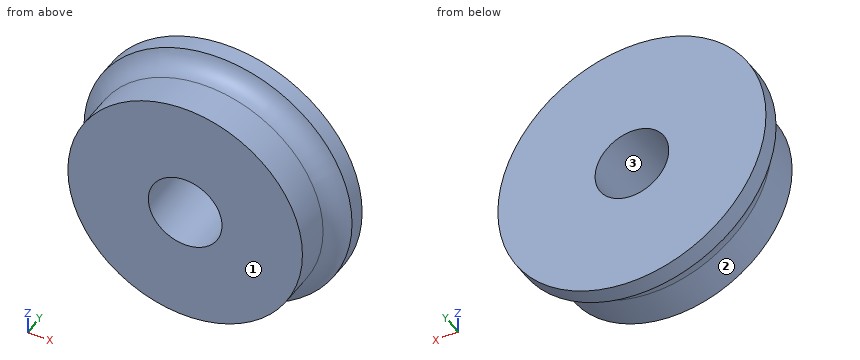
Autodesk Inventor part; units mm, degrees
ref_plane "YZ Plane" through (0, 0, 0) normal (1, 0, 0) x (0, 1, 0)
ref_plane "XZ Plane" through (0, 0, 0) normal (0, 1, 0) x (-1, 0, 0)
ref_plane "XY Plane" through (0, 0, 0) normal (0, 0, 1) x (1, 0, 0)
sketch "Boceto1" plane through (0, 0, 0) normal (0, 1, 0) x (-1, 0, 0)
  circle A0 centre (0, 0) radius 5.25
  dimension "d0" = 10.5
extrude "Extrusión1" add sketch "Boceto1" along normal blind 2.6
sketch "Boceto2" plane through (0, 2.6, 0) normal (0, 1, 0) x (1, 0, 0)
  circle A0 centre (0, 0) radius 6
  dimension "d3" = 12
extrude "Extrusión2" add sketch "Boceto2" along normal blind 0.8
sketch "Boceto3" plane through (0, 3.4, 0) normal (0, 1, 0) x (1, 0, 0)
  circle A0 centre (0, 0) radius 1.65
  dimension "d6" = 3.3
extrude "Extrusión3" cut sketch "Boceto3" against normal through all
fillet "Empalme1" radius 1 1 edges at (5.25, 2.6, 0)
properties part number "RubberSupport"
Model file for the job. Use its own axes, mm. Face numbers are marked on the shaded views. Round coordinates to 2 decimals unless told otherwise and drop trailing zeros. Write each loop counter-clockwise with the first axis right and the second up, starting at its lowest first coordinate (ties: lowest second). Pieces come first, ordered by that corner, then holes. Notation, with made-up numbers: (-38.75, 51.5) - (-27.75, 51.5) arc R23 cw to (-27.75, 68.5) - close; hole circle Ø3 at (-27, 83). An arc over 180 degrees is marked (long way). Use CSV: the item, a comma, the result in double quotes. Start each with the question number.
Item 1: Band-saw the part on A-A (x = 0). Write the cut outline in (y, z), and give its area (3 significant figures).
Item 2: Drill centre lines: L1, parallel to Z at x = 0, y = 0.9; L2, parallel to Z at x = 0, y = 2.7; L3, parallel to X at y = 0.3, z = 0.75. Where is each one in solid material? Low to high. Write a range as [from, to].
Item 3: Band-saw the part on B-B (z = 0). Write the cut outline in (x, y).
Item 4: Band-saw the part on C-C (y = 0.75). Write the cut outline in (x, z).
Item 5: Pin check, flat tips, straight feed: P1, Ø1.5, axis at x = -3, y = 3, coming from the -Z side; P2, Ø5, axis at x = 2, z = 3.5, coming from the -Y side. Stop position of each tip, or through.
Item 6: Two-plate mould, pull along X, no slides. Class the marked faces 1, 2 and 3: released by +X, released by -X, zero draft, split by the parting line, or undercut.
Checked values:
1,outline,"(0, -5.25) - (1.63, -5.25) arc R1 cw to (2.6, -6) - (3.4, -6) - (3.4, -1.65) - (0, -1.65) - close; (0, 1.65) - (3.4, 1.65) - (3.4, 6) - (2.6, 6) arc R1 cw to (1.63, 5.25) - (0, 5.25) - close"
1,area,"26.1 mm²"
2,L1,"z = [-5.25, -1.65], [1.65, 5.25]"
2,L2,"z = [-6, -1.65], [1.65, 6]"
2,L3,"x = [-5.2, -1.47], [1.47, 5.2]"
3,outline,"(-6, 2.6) arc R1 cw to (-5.25, 1.63) - (-5.25, 0) - (-1.65, 0) - (-1.65, 3.4) - (-6, 3.4) - close; (1.65, 0) - (5.25, 0) - (5.25, 1.63) arc R1 cw to (6, 2.6) - (6, 3.4) - (1.65, 3.4) - close"
4,outline,"circle Ø10.5 at (0, 0); hole circle Ø3.3 at (0, 0)"
5,P1,"stops at z = -5.56"
5,P2,"stops at y = 0"
6,face 1,"zero draft"
6,face 2,"split by the parting line"
6,face 3,"undercut"
